For this review, take the finished solid that the model builds, in its own axes (mm). Face numbers are marked on the shaded views. A direction names the side the tool comes from. Give positions to 0.01 mm unless a question says otherwise; leave off trailing zeros. Write each loop counter-clockwise with the first axis right and the second up, starting at its lowest first coordinate (ties: lowest second). Pieces come first, ordered by that corner, then holes. Notation, with made-up numbers: (78, -2.5) -> (128, -2.5) arc R24 ccw to (128, 10.5) -> close; hole circle Ø7 at (-1, -29.75). An arc over 180 degrees is marked (long way). Return JSON: item names as keys, results as strings.
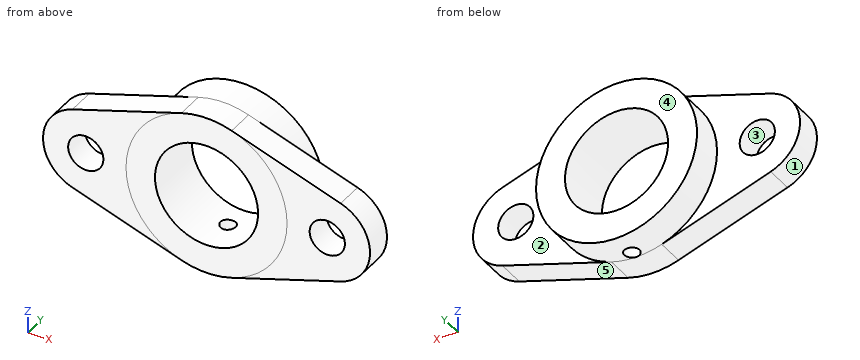
from build123d import *

# Parameters (mm, degrees)
EXTRUDE_2_DEPTH     = 11
SKETCH_2_R          = 7
CUT_EXTRUDE_1_DEPTH = 11
SKETCH_3_R          = 32
EXTRUDE_3_DEPTH     = 24
SKETCH_4_R          = 20.5
CUT_EXTRUDE_2_DEPTH = 25
SKETCH_5_R          = 3
CUT_EXTRUDE_3_DEPTH = 33


with BuildPart() as part:
    # 스케치1 → 보스-돌출2 (new body)
    with BuildSketch(Plane(origin=(0, 0, 0), x_dir=(1, 0, 0), z_dir=(0, 1, 0))):
        with BuildLine():
            Line((-53.3125, 16.148601913), (-10, 30.397368307))
            ThreePointArc((-10, 30.397368307), (0, 32), (10, 30.397368307))
            Line((10, 30.397368307), (53.3125, 16.148601913))
            ThreePointArc((53.3125, 16.148601913), (65, 0), (53.3125, -16.148601913))
            Line((53.3125, -16.148601913), (10, -30.397368307))
            ThreePointArc((10, -30.397368307), (0, -32), (-10, -30.397368307))
            Line((-10, -30.397368307), (-53.3125, -16.148601913))
            ThreePointArc((-53.3125, -16.148601913), (-65, 0), (-53.3125, 16.148601913))
        make_face()
    extrude(amount=EXTRUDE_2_DEPTH)

    # 스케치2 → 컷-돌출1 (cut)
    with BuildSketch(Plane(origin=(0, 0, 0), x_dir=(1, 0, 0), z_dir=(0, 1, 0))):
        with Locations((-48, 0)):
            Circle(SKETCH_2_R)
        with Locations((48, 0)):
            Circle(SKETCH_2_R)
    extrude(amount=CUT_EXTRUDE_1_DEPTH, mode=Mode.SUBTRACT)

    # 스케치3 → 보스-돌출3 (add)
    with BuildSketch(Plane(origin=(0, 0, 0), x_dir=(1, 0, 0), z_dir=(0, 1, 0))):
        Circle(SKETCH_3_R)
    extrude(amount=EXTRUDE_3_DEPTH)

    # 스케치4 → 컷-돌출2 (cut, through all)
    with BuildSketch(Plane(origin=(0, 0, 0), x_dir=(1, 0, 0), z_dir=(0, 1, 0))):
        Circle(SKETCH_4_R)
    extrude(amount=CUT_EXTRUDE_2_DEPTH, mode=Mode.SUBTRACT)

    # 스케치5 → 컷-돌출3 (cut, through all)
    with BuildSketch(Plane.XY):
        with Locations((0, 14)):
            Circle(SKETCH_5_R)
    extrude(amount=-CUT_EXTRUDE_3_DEPTH, mode=Mode.SUBTRACT)


solid = part.part
1. To check wall thickness, follow probe 1 along X at (y, z) = (6, 6); probe 2 along Y at (x, z) = (-35, 2.5); probe 3 along Z at (x, y) = (14.5, 5.5). State the ranges of each line that lie inside material, in increasing order.
Results found:
{"probe 1": "x = -63.91 to -51.61, -44.39 to -19.6, 19.6 to 44.39, 51.61 to 63.91", "probe 2": "y = 0 to 11", "probe 3": "z = -28.92 to -14.49, 14.49 to 28.92"}
2. Add section A-A, the plane z = 0. State the section outline as (x, y) points, plus the area to 3 significant figures.
Results found:
{"outline": "(-65, 0) -> (-55, 0) -> (-55, 11) -> (-65, 11) -> close; (-41, 0) -> (-20.5, 0) -> (-20.5, 24) -> (-32, 24) -> (-32, 11) -> (-41, 11) -> close; (20.5, 0) -> (41, 0) -> (41, 11) -> (32, 11) -> (32, 24) -> (20.5, 24) -> close; (55, 0) -> (65, 0) -> (65, 11) -> (55, 11) -> close", "area": "970 mm²"}
3. Add section D-D, the plane x = -48. State the section outline as (y, z) points.
Results found:
{"outline": "(0, -17.9) -> (11, -17.9) -> (11, -7) -> (0, -7) -> close; (0, 7) -> (11, 7) -> (11, 17.9) -> (0, 17.9) -> close"}
4. For pin 1 (2 mm diameter, centred on y = 19, z = -7, fed in from -X); pin 2 (5 mm diameter, centred on x = -2.5, y = 8, fed in from +Z); pin 3 (10 mm diameter, centred on x = 6.5, y = 16.5, fed in from -Z); pin 4 (16.5 mm diameter, centred on x = 39.5, z = -13, fed in from +Y), all flat-tipped, find the tip position at first contact; note any pin that passes through.
Results found:
{"pin 1": "stops at x = -31.43", "pin 2": "stops at z = 32", "pin 3": "stops at z = -31.96", "pin 4": "stops at y = 11"}
5. The part is to be moulded in two halves that separate along X. For the marked faces 3, 4 and 5, say which applies: +X half, -X half, draft (parallel to the pull), parting line (faces both ways), or undercut.
Results found:
{"face 3": "undercut", "face 4": "draft", "face 5": "+X half"}
6. For the marked faces 1 and 2, list the 3-axis set-ups (+Z, -Z, +X, -X, +Y, -Y) from which the entire face can be reached by the end or side of a thin tool; tool diameter is ignored.
Results found:
{"face 1": "-X, +Y, -Y", "face 2": "+X, +Y"}
7. Add section B-B, the plane x = 0. State the section outline as (y, z) points, plus the area to 3 significant figures.
Results found:
{"outline": "(0, -32) -> (11, -32) -> (11, -20.5) -> (0, -20.5) -> close; (0, 20.5) -> (24, 20.5) -> (24, 32) -> (0, 32) -> close; (17, -32) -> (24, -32) -> (24, -20.5) -> (17, -20.5) -> close", "area": "483 mm²"}
8. Add section C-C, the plane y = 4.75. State the section outline as (x, z) points, plus the area to 3 significant figures.
Results found:
{"outline": "(-53.31, -16.15) -> (-10, -30.4) arc R32 ccw to (10, -30.4) -> (53.31, -16.15) arc R17 ccw to (53.31, 16.15) -> (10, 30.4) arc R32 ccw to (-10, 30.4) -> (-53.31, 16.15) arc R17 ccw to start; hole circle Ø14 at (-48, 0); hole circle Ø41 at (0, 0); hole circle Ø14 at (48, 0)", "area": "4,220 mm²"}
